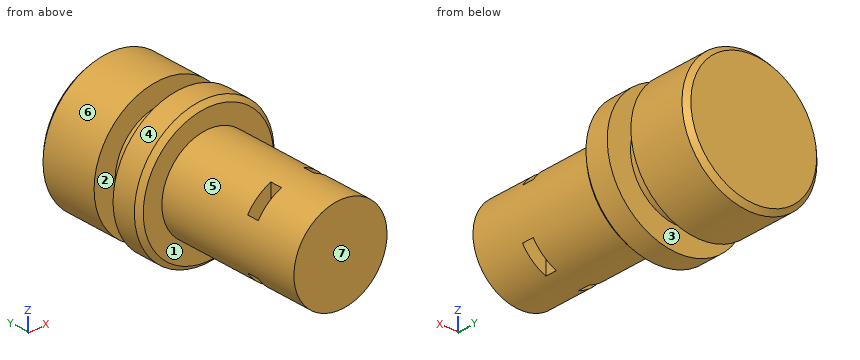
```python
from build123d import *

# Parameters (mm, degrees)
SKETCH_1_R               = 14.5
EXTRUDE_1_DEPTH          = 13
CHAMFER_1_SIZE           = 1
SKETCH_2_R               = 10
EXTRUDE_2_DEPTH          = 42
CUT_EXTRUDE_1_DEPTH      = 47.738634982
CUT_EXTRUDE_1_DEPTH_BACK = 47.738634982
SKETCH_3_W               = 5
SKETCH_3_H               = 2.5
EXTRUDE_3_REACH          = 51.452
SKETCH_5_R               = 1
EXTRUDE_START            = 5
SKETCH_6_R               = 15
EXTRUDE_4_DEPTH          = 6
CHAMFER_3_SIZE           = 1


with BuildPart() as part:
    # Эскиз1 → Бобышка-Вытянуть1 (new body)
    with BuildSketch(Plane(origin=(0, 0, 0), x_dir=(1, 0, 0), z_dir=(0, 1, 0))):
        with Locations(Location((0, 0, 0), (0, 0, 90))):
            Circle(SKETCH_1_R)
    extrude(amount=EXTRUDE_1_DEPTH)

    # Фаска1
    chamfer_1_edges = [part.edges().sort_by_distance(p)[0] for p in [
        (0, 13, 14.5),
    ]]
    chamfer(chamfer_1_edges, length=CHAMFER_1_SIZE)

    # Эскиз2 → Бобышка-Вытянуть2 (add)
    with BuildSketch(Plane.XZ):
        with Locations(Location((0, 0, 0), (0, 0, 90))):
            Circle(SKETCH_2_R)
    extrude(amount=EXTRUDE_2_DEPTH)

    # Эскиз3 → Вырез-Вытянуть1 (cut, two sides: drawn at the far end of the back side and taken through both)
    with BuildSketch(Plane.XY.offset(-CUT_EXTRUDE_1_DEPTH_BACK)):
        with Locations((-6, -30.75)):
            Rectangle(SKETCH_3_W, SKETCH_3_H)
        with Locations((6, -30.75)):
            Rectangle(SKETCH_3_W, SKETCH_3_H)
    extrude(amount=CUT_EXTRUDE_1_DEPTH + CUT_EXTRUDE_1_DEPTH_BACK, mode=Mode.SUBTRACT)

    # Эскиз5 → Бобышка-Вытянуть3 (add, up to next)
    with BuildSketch(Plane(origin=(0, -32, 0), x_dir=(1, 0, 0), z_dir=(0, 1, 0)), mode=Mode.PRIVATE) as extrude_3_sk1:
        with Locations(Location((6, 0, 0), (0, 0, 90))):
            Circle(SKETCH_5_R)
    extrude_3_tool1 = extrude(extrude_3_sk1.sketch, amount=EXTRUDE_3_REACH, mode=Mode.PRIVATE) - part.part
    extrude_3 = extrude_3_tool1.solids().sort_by_distance((6, -32, 0))[0]
    add(extrude_3)

    # Зеркальное отражение1: Бобышка-Вытянуть3 across plane
    add(extrude_3.mirror(Plane(origin=(0, 0, 0), x_dir=(0, 0, 1), z_dir=(1, 0, 0))))

    # Эскиз6 → Бобышка-Вытянуть4 (add)
    with BuildSketch(Plane.XZ.offset(EXTRUDE_START)):
        with Locations(Location((0, 0, 0), (0, 0, 270))):
            Circle(SKETCH_6_R)
    extrude(amount=EXTRUDE_4_DEPTH)

    # Фаска3
    chamfer_3_edges = [part.edges().sort_by_distance(p)[0] for p in [
        (0, -11, 15),
    ]]
    chamfer(chamfer_3_edges, length=CHAMFER_3_SIZE)


solid = part.part
```
Geometry check sheet. Reference: the model listing, model coordinates, mm. Face numbers are marked on the shaded views. A direction names the side the tool comes from. Coordinates: 2 decimals unless noted, no trailing zeros. Loops run counter-clockwise (first coordinate to the right, second up) from the corner with the lowest first, then second, coordinate; pieces in that order, holes last.
Item 1: Release check for a two-part mould opening along Y. For the marked faces 1, 2, 3 and 4 record: released by +Y, released by -Y, zero draft, split by the parting line, or undercut.
Item 2: Go/stop test with flat-tipped pins: pin 1 Ø10 at (x, y) = (3, -14.5) entering from -Z; pin 2 Ø3 at (y, z) = (-8.5, 7) entering from +X; pin 3 Ø1 at (y, z) = (-27, -11) entering from -X; pin 4 Ø1.2 at (y, z) = (-30, 2.5) entering from -X. Record where each tip stops, or that it passes through.
Item 3: Access from +Z, -Z, +X, -X, +Y, -Y to the whole of each face (thin tool, end or side, straight path). Record for the marked faces 5, 6 and 7.
Item 4: Thickness scan on line 1 (Y direction, x = -4.75, z = 0.75); line 2 (Y direction, x = -8.5, z = 10); line 3 (X direction, y = -31, z = -4.75). Record the ranges inside material, lowest first.
Item 5: Sectioned sample at C-C, the plane y = -26.5. Record the boundary of the cut face in (x, z), then the cut area to 3 significant figures.
Item 6: Sectioned sample at A-A, the plane z = 0. Count the separate pieces of the cut face and the enclosed holes in it, then the cut area to 3 significant figures.
Item 7: Sectioned sample at B-B, the plane y = 5. Record the boundary of the cut face in (x, z).
Check result:
1. face 1: released by -Y
1. face 2: undercut
1. face 3: undercut
1. face 4: zero draft
2. pin 1: stops at z = -14.98
2. pin 2: stops at x = 13.96
2. pin 3: passes through
2. pin 4: stops at x = -9.82
3. face 5: -Y
3. face 6: +Y
3. face 7: +Z, -Z, +X, -X, -Y
4. line 1: y = -42 to -32, -29.5 to 13
4. line 2: y = -11 to -5, 0 to 13
4. line 3: x = -8.8 to -8.5, -3.5 to 3.5, 8.5 to 8.8
5. outline: circle Ø20 at (0, 0)
5. area: 314 mm2
6. separate pieces: 1
6. enclosed holes: 4
6. area: 1,260 mm2
7. outline: circle Ø29 at (0, 0)
